Autodesk Inventor part; units mm, degrees
ref_plane "YZ Plane" through (0, 0, 0) normal (1, 0, 0) x (0, 1, 0)
ref_plane "XZ Plane" through (0, 0, 0) normal (0, 1, 0) x (-1, 0, 0)
ref_plane "XY Plane" through (0, 0, 0) normal (0, 0, 1) x (1, 0, 0)
sketch "Sketch1" plane through (0, 0, 0) normal (0, 0, 1) x (1, 0, 0)
  line L0 (-6.35, -3.6662) -> (-6.35, 3.6662)
  line L1 (-6.35, 3.6662) -> (0, 7.3323)
  line L2 (0, 7.3323) -> (6.35, 3.6662)
  line L3 (6.35, 3.6662) -> (6.35, -3.6662)
  line L4 (6.35, -3.6662) -> (0, -7.3323)
  line L5 (0, -7.3323) -> (-6.35, -3.6662)
  point P0 (0, 0)
  point P1 (0, 0)
  dimension "Size" = 12.7
extrude "Extrusion1" add sketch "Sketch1" along normal mid plane 166.9034
sketch "Sketch3" plane through (0, 0, 83.4517) normal (0, 0, 1) x (1, 0, 0)
  line L0 (-6.35, 3.6662) -> (0, 7.3323) construction
  line L1 (0, 7.3323) -> (6.35, 3.6662) construction
  line L2 (6.35, 3.6662) -> (6.35, -3.6662) construction
  line L3 (6.35, -3.6662) -> (0, -7.3323) construction
  line L4 (0, -7.3323) -> (-6.35, -3.6662) construction
  line L5 (-6.35, -3.6662) -> (-6.35, 3.6662) construction
  point P0 (0, 0)
hole "Hole1" at (0, 0, 83.4517) direction (0, 0, -1) diameter 5.1054 end through all
sketch "Sketch4" plane through (0, 0, 83.4517) normal (0, 0, 1) x (1, 0, 0)
  circle A0 centre (0, 0) radius 2.5527 construction
  line L0 (-6.35, 3.6662) -> (0, 7.3323) construction
  line L1 (0, 7.3323) -> (6.35, 3.6662) construction
  line L2 (6.35, 3.6662) -> (6.35, -3.6662) construction
  line L3 (6.35, -3.6662) -> (0, -7.3323) construction
  line L4 (0, -7.3323) -> (-6.35, -3.6662) construction
  line L5 (-6.35, -3.6662) -> (-6.35, 3.6662) construction
  circle A1 centre (0, 0) radius 6.8771
  circle A2 centre (0, 0) radius 8.89
  dimension "thunder" = 13.7541
  dimension "d16" = 17.78
extrude "Extrusion3" cut sketch "Sketch4" against normal through all
equation "\"bearing\" = 25.4"
properties part number "GP3-005" material "Aluminum 6061"
Input: part model. Units: mm. Frame: model coordinates. Round coordinates to 2 decimals unless told otherwise and drop trailing zeros. Loops run counter-clockwise (first coordinate to the right, second up) from the corner with the lowest first, then second, coordinate; pieces in that order, holes last. Notation, with made-up numbers: (-1, 7.5) -> (32, 7.5) arc R36 cw to (32, 43.5) -> close; hole circle Ø6 at (14.25, -6.75). An arc over 180 degrees is marked (long way). Answer as a JSON object with one key per item and string values. Group by question number.
1) Ray query, L1, parallel to X at y = 0, z = 31; L2, parallel to Y at x = 0, z = -45.5; L3, parallel to Y at x = 3.25, z = 29.5. Return the intervals inside material, ascending.
2) Section query A-A on z = -4. Output: boundary loops of the cut face in (x, y), plus the area to 3 significant figures.
3) Pin query (flat end, axial travel): pin 1 (3 mm diameter, centred on x = 2.5, z = -49, fed in from +Y); pin 2 (1 mm diameter, centred on x = 1, z = 28, fed in from +Y); pin 3 (2 mm diameter, centred on x = -4, z = 66, fed in from +Y); pin 4 (3 mm diameter, centred on x = 0, y = 0, fed in from -Z). Return the tip coordinate at first contact, or that it passes through.
4) Section query B-B on y = 0. Output: boundary loops of the cut face in (x, z).
5) Draft query along X for faces 1 (the flat face through (3.21, -5.48, -1.17)), 2 (the flat face through (-3, 0, 83.452)), 3 (the cylindrical face through (-0.767, -2.435, -1.168)). Return one class per face: +X half, -X half, draft (parallel to the pull), parting line (faces both ways), or undercut.
Reply:
{
 "1": {"L1": "x = -6.35 to -2.55, 2.55 to 6.35", "L2": "y = -6.88 to -2.55, 2.55 to 6.88", "L3": "y = -5.46 to 5.46"},
 "2": {"outline": "(-6.35, -2.64) arc R6.88 ccw to (-5.46, -4.18) -> (-0.89, -6.82) arc R6.88 ccw to (0.89, -6.82) -> (5.46, -4.18) arc R6.88 ccw to (6.35, -2.64) -> (6.35, 2.64) arc R6.88 ccw to (5.46, 4.18) -> (0.89, 6.82) arc R6.88 ccw to (-0.89, 6.82) -> (-5.46, 4.18) arc R6.88 ccw to (-6.35, 2.64) -> close; hole circle Ø5.11 at (0, 0)", "area": "117 mm2"},
 "3": {"pin 1": "stops at y = 6.75", "pin 2": "stops at y = 6.86", "pin 3": "stops at y = 5.6", "pin 4": "passes through"},
 "4": {"outline": "(-6.35, -83.45) -> (-2.55, -83.45) -> (-2.55, 83.45) -> (-6.35, 83.45) -> close; (2.55, -83.45) -> (6.35, -83.45) -> (6.35, 83.45) -> (2.55, 83.45) -> close"},
 "5": {"face 1": "+X half", "face 2": "draft", "face 3": "undercut"}
}
